Geometry check sheet. Reference: the model listing, model coordinates, mm. A direction names the side the tool comes from. Round coordinates to 2 decimals unless told otherwise and drop trailing zeros. Order: outer loops, then holes, each group sorted by start corner. A loop starts at its lowest first (then second) coordinate and runs counter-clockwise, first axis right, second up. Notation, with made-up numbers: (-30, 3.25) - (19, 3.25) arc R29 cw to (19, 30.25) - close; hole circle Ø9 at (28, 74.25). An arc over 180 degrees is marked (long way). One line per question, with ' | ' between items. Start each with the question number.
Q1. Sectioned sample at D-D, the plane x = -44. Enter the section's corners in (y, z), then the cut area to 3 significant figures.
Q2. Sectioned sample at B-B, the plane x = 8.5. Enter the section's corners in (y, z), then the cut area to 3 significant figures.
Q3. Sectioned sample at C-C, the plane y = 1.05. Enter the section's corners in (x, z) (1 decimal).
Q4. Material ranges on line 1 along X through (y, z) = (0.7, 0); line 2 along X through (y, z) = (1.9, -13); line 3 along Z through (x, y) = (0, 0.7), recorded low to high.
Q5. Sectioned sample at A-A, the plane z = 0. Enter the section's corners in (x, y).
Q6. Gauge pin test, flat end, axial feed: P1, Ø1.5, axis at x = 48, y = 0.5, coming from the +Z side. Record the tip position at first contact, or that the pin passes through.
Q7. Tool access check on faces 1 (the face through (-49.28, 1.48, 59.14)), 2 (the face through (-53, 0, 47)). Record the directions out of +Z, -Z, +X, -X, +Y, -Y that give a thin tool (end or side, any length) a straight path to the whole face; none if there is none.
Q8. Mould release check, pull along X, two halves, no side actions. Record for faces 3 (the face through (-60.82, 1.48, 66.34)), 4 (the face through (43.09, 1.48, 67.62)), 5 (the face through (-53, 3, 47)): +X half, -X half, draft (parallel to the pull), parting line (faces both ways), or undercut.
Autodesk Inventor part; units mm, degrees
ref_plane "YZ Plane" through (0, 0, 0) normal (1, 0, 0) x (0, 1, 0)
ref_plane "XZ Plane" through (0, 0, 0) normal (0, 1, 0) x (-1, 0, 0)
ref_plane "XY Plane" through (0, 0, 0) normal (0, 0, 1) x (1, 0, 0)
sketch "Sketch1" plane through (0, 0, 0) normal (0, 1, 0) x (-1, 0, 0)
  circle A0 centre (0, 0) radius 70.5
  circle A1 centre (0, 0) radius 90
  line L0 (90, 0) -> (70.5, 0)
  line L1 (-90, 0) -> (-70.5, 0)
  line L2 (0, 0) -> (-70.5, 0) construction
  line L3 (0, 70.5) -> (0, 0) construction
  line L4 (0, 90) -> (0, 70.5)
  line L5 (-70.5, 0) -> (-90, 0)
  line L6 (-74.25, 7) -> (-86.25, 7)
  line L7 (-86.25, 7) -> (-83.7022, 0)
  line L8 (-74.25, 7) -> (-76.7978, 0)
  line L9 (-80.25, 0) -> (-80.25, 7) construction
  line L10 (-55.5838, 59.7031) -> (-30.242, 75.7591)
  line L11 (-30.242, 75.7591) -> (-28.5294, 73.056)
  line L12 (-28.5294, 73.056) -> (-53.8711, 57)
  line L13 (-53.8711, 57) -> (-55.5838, 59.7031)
  line L14 (-55.5838, 59.7031) -> (-28.5294, 73.056) construction
  line L15 (-30.242, 75.7591) -> (-53.8711, 57) construction
  circle A2 centre (0, 0) radius 80 construction
  line L16 (-73.9574, -34.414) -> (-81.3965, -5.351)
  line L17 (-70.8573, -33.6205) -> (-73.9574, -34.414)
  line L18 (-78.2964, -4.5575) -> (-70.8573, -33.6205)
  line L19 (-81.3965, -5.351) -> (-78.2964, -4.5575)
  line L20 (9.8756, -80.9722) -> (-20.0638, -79.0662)
  line L21 (10.0789, -77.7786) -> (9.8756, -80.9722)
  line L22 (-19.8605, -75.8727) -> (10.0789, -77.7786)
  line L23 (-20.0638, -79.0662) -> (-19.8605, -75.8727)
  line L24 (80.0608, -15.6295) -> (68.9964, -43.5146)
  line L25 (77.0864, -14.4493) -> (80.0608, -15.6295)
  line L26 (66.022, -42.3344) -> (77.0864, -14.4493)
  line L27 (68.9964, -43.5146) -> (66.022, -42.3344)
  line L28 (0, 0) -> (-63.6396, -63.6396) construction
  line L29 (0, 0) -> (-60.8031, -66.355)
  line L30 (0, 0) -> (-66.355, -60.8031)
  line L31 (39.6047, 71.3126) -> (62.7059, 52.1727)
  line L32 (37.5631, 68.8485) -> (39.6047, 71.3126)
  line L33 (60.6643, 49.7086) -> (37.5631, 68.8485)
  line L34 (62.7059, 52.1727) -> (60.6643, 49.7086)
  point P0 (80.25, 0)
  point P1 (-80.25, 0)
  point P2 (-42.0566, 66.3795)
  point P3 (-15.2947, 78.5243)
  point P4 (-54.7275, 58.3516)
  point P5 (-29.3857, 74.4075)
  point P6 (-72.4073, -34.0173)
  point P7 (-79.8464, -4.9543)
  point P8 (9.9773, -79.3754)
  point P9 (-19.9621, -77.4694)
  point P10 (78.5736, -15.0394)
  point P11 (67.5092, -42.9245)
  point P12 (-76.7978, 0)
  point P13 (-83.7022, 0)
  point P14 (38.5839, 70.0805)
  point P15 (61.6851, 50.9406)
  point P16 (-51.9781, -47.6291)
  point P17 (-47.6291, -51.9781)
  dimension "d1" = 180
  dimension "d0" = 141
  dimension "d4" = 90
  dimension "d5" = 7
  dimension "d6" = 70
  dimension "d8" = 12
  dimension "d13" = 3.2
  dimension "d14" = 30
  dimension "d15" = 50
  dimension "d20" = 160
  dimension "d27" = 360
  dimension "d29" = 45
  dimension "d32" = 5
  dimension "d33" = 2.5
extrude "Extrusion1" add sketch "Sketch1" along normal blind 3 contours L0 A1 L29 A0 | A0 L4 A1 L0 | A0 L1 L8 L6 L7 A1 L4 | A0 L30 A1 L1 | L1 L7 L6 L8
equation "\"d33\" = 0.5 * d32"
properties part number "D14_CM_CIRCULO" material "MDF Medium Density Fiberboard"
Determined:
1) outline: (0, -78.51) - (3, -78.51) - (3, -55.08) - (0, -55.08) - close; (0, 55.08) - (3, 55.08) - (3, 63.52) - (0, 63.52) - close; (0, 67.67) - (3, 67.67) - (3, 78.51) - (0, 78.51) - close | area: 128 mm2
2) outline: (0, -89.6) - (3, -89.6) - (3, -79.8) - (0, -79.8) - close; (0, -76.6) - (3, -76.6) - (3, -69.99) - (0, -69.99) - close; (0, 69.99) - (3, 69.99) - (3, 89.6) - (0, 89.6) - close | area: 108 mm2
3) outline: (47.6, -52) arc R70.5 cw (long way) to (52, -47.6) - (66.4, -60.8) arc R90 ccw (long way) to (60.8, -66.4) - close; hole (-80.1, -15.6) - (-69, -43.5) - (-66, -42.3) - (-77.1, -14.4) - close; hole (-62.7, 52.2) - (-60.7, 49.7) - (-37.6, 68.8) - (-39.6, 71.3) - close; hole (-10.1, -77.8) - (-9.9, -81) - (20.1, -79.1) - (19.9, -75.9) - close; hole (28.5, 73.1) - (53.9, 57) - (55.6, 59.7) - (30.2, 75.8) - close; hole (70.9, -33.6) - (74, -34.4) - (81.4, -5.4) - (78.3, -4.6) - close
4) line 1: x = -90 to -70.5, 70.5 to 90 | line 2: x = -89.06 to -69.29, 69.29 to 76.14, 79.44 to 89.06 | line 3: z = -90 to -80.34, -77.14 to -70.5, 70.5 to 90
5) outline: (-90, 0) - (-70.5, 0) - (-70.5, 3) - (-90, 3) - close; (70.5, 0) - (90, 0) - (90, 3) - (70.5, 3) - close
6) P1: stops at z = 76.6
7) face 1: +Y, -Y | face 2: +Z, -Z, +X, -X, -Y
8) face 3: parting line | face 4: undercut | face 5: draft
